Verification items for the finished model (mm, model axes). A direction names the side the tool comes from. Give positions to 0.01 mm unless a question says otherwise; leave off trailing zeros. Loops run counter-clockwise (first coordinate to the right, second up) from the corner with the lowest first, then second, coordinate; pieces in that order, holes last. Notation, with made-up numbers: M 20,44.25 L 58,44.25 A23 ccw 58,59.25 Z; hole C -11,67.25 d7. An arc over 180 degrees is marked long. Answer in a Markdown table with one row per item.
```python
from build123d import *

# Parameters (mm, degrees)
F0_R     = 6
F0_R_2   = 3
F1_DEPTH = 2
F0_R_3   = 1.5
F2_DEPTH = 4
F4_DEPTH = 30.5
F5_SIZE  = 2.99999


# Not quite as in the source:
# - a fillet or chamfer is up to 0.001 mm smaller than in the source, because OpenCascade refuses the exact size


with BuildPart() as f1:
    # F0 (on Top) → F1 (new body)
    with BuildSketch(Plane.XY):
        Circle(F0_R)
        Circle(F0_R_2, mode=Mode.SUBTRACT)
    extrude(amount=F1_DEPTH)



with BuildPart() as f2:
    # F0 (on Top) → F2 (new body)
    with BuildSketch(Plane.XY):
        Circle(F0_R_3)
    extrude(amount=F2_DEPTH)


with BuildPart() as f1_1:
    add(f1.part)

    add(f2.part)  # F4 merges F2
    # F0 (on Top) → F4 (join)
    with BuildSketch(Plane.XY):
        Circle(F0_R_2)
        Circle(F0_R_3, mode=Mode.SUBTRACT)
    extrude(amount=F4_DEPTH)

    # F5 (size 3 in the source; OpenCascade refuses exactly that, so slightly less here)
    f5_edges = [f1_1.edges().sort_by_distance(p)[0] for p in [
        (-3, 0, 2),
    ]]
    chamfer(f5_edges, length=F5_SIZE)


solid = f1_1.part
```
Item 1: Sectioned sample at A-A (z = 6.5). Record the cut outline in (x, y).
Reported:
| item | result |
|---|---|
| outline | C 0,0 d6; hole C 0,0 d3 |
Item 2: Scan lines: L1, parallel to Y at x = 0, z = 22; L2, parallel to X at y = 0.25, z = 27.5; L3, parallel to X at y = 0.5, z = 24. Record each from-to range of solid material in increasing order. Write a range as [from, to].
Reported:
| item | result |
|---|---|
| L1 | y = [-3, -1.5], [1.5, 3] |
| L2 | x = [-2.99, -1.48], [1.48, 2.99] |
| L3 | x = [-2.96, -1.41], [1.41, 2.96] |
Item 3: Go/stop test with flat-tipped pins: pin 1 (5 mm diameter, centred on x = -2, z = 26, fed in from +Y); pin 2 (3 mm diameter, centred on y = 2, z = 9.5, fed in from +X); pin 3 (1.5 mm diameter, centred on y = -2, z = 17, fed in from +X). Record where each tip stops, or that it passes through.
Reported:
| item | result |
|---|---|
| pin 1 | stops at y = 3 |
| pin 2 | stops at x = 2.96 |
| pin 3 | stops at x = 2.73 |
Item 4: Release check for a two-part mould opening along Y. For faces 1 (the flat face through (1.3, -1.3, 30.5)), 2 (the conical face through (-0.691, -3.112, 4.812)), 3 (the flat face through (0, 0, 4)) record: released by +Y, released by -Y, zero draft, split by the parting line, or undercut.
Reported:
| item | result |
|---|---|
| face 1 | zero draft |
| face 2 | split by the parting line |
| face 3 | undercut |
Item 5: Tool access check on faces 4 (the cylindrical face through (-6, 0, 1)), 5 (the cylindrical face through (-1.5, 0.07, 17.06)). Record the directions out of +Z, -Z, +X, -X, +Y, -Y that give a thin tool (end or side, any length) a straight path to the whole face; none if there is none.
Reported:
| item | result |
|---|---|
| face 4 | +Z, -Z |
| face 5 | +Z |
